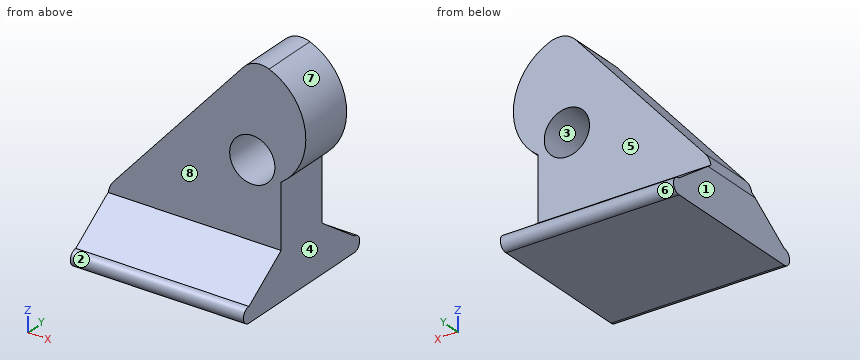
from build123d import *

# Parameters (mm, degrees)
SKETCH1_R               = 2.4892
BOSS_EXTRUDE1_DEPTH     = 6.35
BOSS_EXTRUDE2_START     = -6.35
BOSS_EXTRUDE2_DEPTH     = 19.05
BOSS_EXTRUDE2_START_2   = -6.555460136
BOSS_EXTRUDE2_2_DEPTH   = 19.460920272
BOSS_EXTRUDE2_START_3   = -10
BOSS_EXTRUDE2_3_DEPTH   = 3.65
CUT_EXTRUDE1_DEPTH      = 27.910448217
CUT_EXTRUDE1_DEPTH_BACK = 27.910448217
SKETCH3_W               = 2.179354936
SKETCH3_H               = 6.35
CUT_EXTRUDE2_DEPTH      = 31.98795935
CUT_EXTRUDE2_DEPTH_BACK = 31.98795935
BOSS_EXTRUDE4_START     = -6.35
SKETCH8_R               = 2.4892
BOSS_EXTRUDE4_DEPTH     = 6.35
CUT_EXTRUDE3_DEPTH      = 27.585891059
CUT_EXTRUDE3_DEPTH_BACK = 27.585891059
SKETCH7_R               = 2.4892
CUT_EXTRUDE4_DEPTH      = 27.585891059
CUT_EXTRUDE4_DEPTH_BACK = 27.585891059
FILLET1_R               = 2.54


with BuildPart() as part:
    # Sketch1 → Boss-Extrude1 (new body)
    with BuildSketch(Plane(origin=(0, 0, 0), x_dir=(1, 0, 0), z_dir=(0, 1, 0))):
        with BuildLine():
            Line((9.525, -17.889269346), (-0.578271622, -16.817120786))
            Line((-0.578271622, -16.817120786), (-6.35, 0))
            Line((-6.35, 0), (12.7, 0))
            Line((12.7, 0), (12.7, -6.35))
            ThreePointArc((12.7, -6.35), (15.186560179, -13.240601753), (9.525, -17.889269346))
        make_face()
        with Locations(Location((9.525, -11.43, 0), (0, 0, 270))):
            Circle(SKETCH1_R, mode=Mode.SUBTRACT)
    extrude(amount=BOSS_EXTRUDE1_DEPTH)

    # Boss-Extrude2: read off the stored shape, not the designer's step
    # Boss-Extrude2 outline → Boss-Extrude2 (add)
    with BuildSketch(Plane.YZ.offset(BOSS_EXTRUDE2_START)):
        with BuildLine():
            ThreePointArc((11.551615481, -6.35), (12.905510296, -4.996105185), (11.551615481, -3.642210371))
            Line((11.551615481, -3.642210371), (6.35, 0))
            Line((6.35, 0), (0, 0))
            Line((0, 0), (-5.201615481, -3.642210371))
            ThreePointArc((-5.201615481, -3.642210371), (-6.555510296, -4.996105185), (-5.201615481, -6.35))
            Line((-5.201615481, -6.35), (11.551615481, -6.35))
        make_face()
    extrude(amount=BOSS_EXTRUDE2_DEPTH)

    # Boss-Extrude2 2 outline → Boss-Extrude2 2 (add)
    with BuildSketch(Plane(origin=(0, 0, 0), x_dir=(1, 0, 0), z_dir=(0, 1, 0)).offset(BOSS_EXTRUDE2_START_2)):
        Polygon((-8.529354936, 6.35), (-6.35, 0), (-6.35, 6.35), align=None)
    extrude(amount=BOSS_EXTRUDE2_2_DEPTH)

    # Boss-Extrude2 3 outline → Boss-Extrude2 3 (cut)
    with BuildSketch(Plane.YZ.offset(BOSS_EXTRUDE2_START_3)):
        with BuildLine():
            Line((12.905460136, 0), (6.35, 0))
            Line((6.35, 0), (11.551615481, -3.642210371))
            ThreePointArc((11.551615481, -3.642210371), (12.504834401, -4.034645431), (12.905460136, -4.984450993))
            Line((12.905460136, -4.984450993), (12.905460136, 0))
        make_face()
        with BuildLine():
            ThreePointArc((12.905460136, -5.007759378), (12.504834401, -5.95756494), (11.551615481, -6.35))
            Line((11.551615481, -6.35), (12.905460136, -6.35))
            Line((12.905460136, -6.35), (12.905460136, -5.007759378))
        make_face()
        with BuildLine():
            Line((0, 0), (-6.555460136, 0))
            Line((-6.555460136, 0), (-6.555460136, -4.984450993))
            ThreePointArc((-6.555460136, -4.984450993), (-6.154834401, -4.034645431), (-5.201615481, -3.642210371))
            Line((-5.201615481, -3.642210371), (0, 0))
        make_face()
        with BuildLine():
            ThreePointArc((-5.201615481, -6.35), (-6.154834401, -5.95756494), (-6.555460136, -5.007759378))
            Line((-6.555460136, -5.007759378), (-6.555460136, -6.35))
            Line((-6.555460136, -6.35), (-5.201615481, -6.35))
        make_face()
    extrude(amount=BOSS_EXTRUDE2_3_DEPTH, mode=Mode.SUBTRACT)

    # Sketch3 → Cut-Extrude1 (cut, two sides: drawn at the far end of the back side and taken through both)
    with BuildSketch(Plane.XZ.offset(-CUT_EXTRUDE1_DEPTH_BACK)):
        with Locations((-7.439677468, -3.175)):
            Rectangle(SKETCH3_W, SKETCH3_H)
    extrude(amount=CUT_EXTRUDE1_DEPTH + CUT_EXTRUDE1_DEPTH_BACK, mode=Mode.SUBTRACT)

    # Sketch4 → Cut-Extrude2 (cut, two sides: drawn at the far end of the back side and taken through both)
    with BuildSketch(Plane.ZY.offset(6.35).offset(-CUT_EXTRUDE2_DEPTH_BACK)):
        with BuildLine():
            ThreePointArc((-5.842, -5.006022622), (-4.983704134, -5.864318488), (-4.125408268, -5.006022622))
            Line((-4.125408268, -5.006022622), (-0.620153491, 0))
            Line((-0.620153491, 0), (0, 0))
            Line((0, 0), (-3.642210371, -5.201615481))
            ThreePointArc((-3.642210371, -5.201615481), (-4.996105185, -6.555510296), (-6.35, -5.201615481))
            Line((-6.35, -5.201615481), (-6.35, 11.551615481))
            ThreePointArc((-6.35, 11.551615481), (-4.996105185, 12.905510296), (-3.642210371, 11.551615481))
            Line((-3.642210371, 11.551615481), (0, 6.35))
            Line((0, 6.35), (-0.620153491, 6.35))
            Line((-0.620153491, 6.35), (-4.125408268, 11.356022622))
            ThreePointArc((-4.125408268, 11.356022622), (-4.983704134, 12.214318488), (-5.842, 11.356022622))
            Line((-5.842, 11.356022622), (-5.842, -5.006022622))
        make_face()
    extrude(amount=CUT_EXTRUDE2_DEPTH + CUT_EXTRUDE2_DEPTH_BACK, mode=Mode.SUBTRACT)

    # Sketch8 → Boss-Extrude4 (add)
    with BuildSketch(Plane(origin=(0, 6.35, 0), x_dir=(1, 0, 0), z_dir=(0, 1, 0)).offset(BOSS_EXTRUDE4_START)):
        with Locations((9.525, -11.43)):
            Circle(SKETCH8_R)
    extrude(amount=BOSS_EXTRUDE4_DEPTH)

    # Sketch7 → Cut-Extrude3 (cut, two sides: drawn at the far end of the back side and taken through both)
    with BuildSketch(Plane(origin=(0, 6.35, 0), x_dir=(1, 0, 0), z_dir=(0, 1, 0)).offset(-CUT_EXTRUDE3_DEPTH_BACK)):
        with Locations(Location((9.525, -7.634846509, 0), (0, 0, 270))):
            Circle(SKETCH7_R)
    extrude(amount=CUT_EXTRUDE3_DEPTH + CUT_EXTRUDE3_DEPTH_BACK, mode=Mode.SUBTRACT)

    # Sketch9 → Cut-Extrude4 (cut, two sides: drawn at the far end of the back side and taken through both)
    with BuildSketch(Plane(origin=(0, 6.35, 0), x_dir=(1, 0, 0), z_dir=(0, 1, 0)).offset(-CUT_EXTRUDE4_DEPTH_BACK)):
        Polygon((9.525, -17.889269346), (-6.35, 0), (-0.578271622, -16.817120786), align=None)
    extrude(amount=CUT_EXTRUDE4_DEPTH + CUT_EXTRUDE4_DEPTH_BACK, mode=Mode.SUBTRACT)

    # Fillet1
    fillet1_edges = [part.edges().sort_by_distance(p)[0] for p in [
        (9.525, 3.175, 17.889269346),
        (-6.35, 3.175, 0),
    ]]
    fillet(fillet1_edges, radius=FILLET1_R)


solid = part.part
Geometry check sheet. Reference: the model listing, model coordinates, mm. Face numbers are marked on the shaded views. A direction names the side the tool comes from. Give positions to 0.01 mm unless a question says otherwise; leave off trailing zeros. Write each loop counter-clockwise with the first axis right and the second up, starting at its lowest first coordinate (ties: lowest second). Pieces come first, ordered by that corner, then holes. Notation, with made-up numbers: M -31.75,16 L 3.25,16 A26 ccw 3.25,36 Z; hole C -40,73.5 d10. An arc over 180 degrees is marked long. Answer as CSV lines item,"result". Start each with the question number.
Q1. Release check for a two-part mould opening along X. For the marked faces 1, 2 and 3 record: pulls with the +X half, pulls with the -X half, needs draft (parallel to the pull), parting line crosses it, or undercut.
Q2. Section check D-D, the plane y = 7.75. Record the cut outline in (x, z).
Q3. Section check A-A, the plane z = 6. Record the cut outline in (x, y), then the cut area to 3 significant figures.
Q4. Material ranges on L1, parallel to X at y = 8, z = -4.5; L2, parallel to Y at x = 2, z = -0.25; L3, parallel to X at y = 4.5, z = 0, recorded low to high.
Q5. Section check C-C, the plane x = 3. Record the cut outline in (y, z).
Q6. Go/stop test with flat-tipped pins: pin 1 (5.5 mm diameter, centred on x = 9, z = 9.5, fed in from -Y); pin 2 (4 mm diameter, centred on x = 9.52, z = 7.63, fed in from -Y); pin 3 (1 mm diameter, centred on x = 1, z = 3.5, fed in from +Y); pin 4 (8 mm diameter, centred on x = 4.5, z = 2.5, fed in from +Y). Record where each tip stops, or that it passes through.
Q7. Tool access check on the marked faces 4, 5, 6, 7 and 8. Record the directions out of +Z, -Z, +X, -X, +Y, -Y that give a thin tool (end or side, any length) a straight path to the whole face; none if there is none.
Geometry says:
1,face 1,"pulls with the -X half"
1,face 2,"needs draft"
1,face 3,"undercut"
2,outline,"M -6.35,-5.84 L 12.7,-5.84 L 12.7,-1.6 L -6.35,-1.6 Z"
3,outline,"M -1.03,0 L 7.65,0 L 7.65,6.35 L -1.03,6.35 Z; M 11.4,0 L 12.7,0 L 12.7,6.35 L 11.4,6.35 Z"
3,area,"63.3 mm^2"
4,L1,"-6.35 to 12.7"
4,L2,"0 to 6.35"
4,L3,"-6.16 to 12.7"
5,outline,"M -5.01,-5.84 L 11.36,-5.84 A0.86 ccw 11.36,-4.13 L 6.35,-0.62 L 6.35,10.54 L 0,10.54 L 0,-0.62 L -5.01,-4.13 A0.86 ccw Z"
6,pin 1,"y = 0"
6,pin 2,"through"
6,pin 3,"y = 6.35"
6,pin 4,"y = 7.61"
7,face 4,"-Z, +X, +Y, -Y"
7,face 5,"+Z, +X, -X, +Y"
7,face 6,"+X, -X, +Y"
7,face 7,"+X, +Y, -Y"
7,face 8,"+Z, +X, -X, -Y"
